```python
from build123d import *

# Parameters (mm, degrees)
F0_W      = 50.8
F0_H      = 76.2
F1_DEPTH  = 7.62
F2_R      = 18.7529717457
F3_DEPTH  = 5.08
F4_R      = 5.07999
F7_DEPTH  = 2.54
F8_W      = 50.2787431046
F8_H      = 6.6451809329
F9_DEPTH  = 2.286
F10_W     = 73.914
F10_H     = 6.6451809329
F11_DEPTH = 2.286
F12_W     = 48.514
F12_H     = 6.6451809329
F13_DEPTH = 2.286
F14_R     = 3.4596539052
F15_DEPTH = 25.4


# Not quite as in the source:
# - a fillet or chamfer is up to 0.001 mm smaller than in the source, because OpenCascade refuses the exact size


with BuildPart() as f1:
    # F0 (on Top) → F1 (new body)
    with BuildSketch(Plane.XY):
        with Locations((0.3819083795, -6.0587156958)):
            Rectangle(F0_W, F0_H)
    extrude(amount=F1_DEPTH)

    # F2 (on face) → F3 (join)
    with BuildSketch(Plane.XY.offset(7.62)):
        Circle(F2_R)
    extrude(amount=F3_DEPTH)

    # F4 (radius 5.08 in the source; OpenCascade refuses exactly that, so slightly less here)
    f4_edges = [f1.edges().sort_by_distance(p)[0] for p in [
        (-18.752972, 0, 12.7),
    ]]
    fillet(f4_edges, radius=F4_R)

    # F5 (on face) + F6 (on face) → F7 (join)
    with BuildSketch(Plane.XY.offset(7.62)):
        with BuildLine():
            ThreePointArc((-17.8012941845, -5.8981246722), (-18.7253311698, -1.0178024727), (-18.33570835, 3.9339228004))
            Line((-18.33570835, 3.9339228004), (-25.0180916205, 0.604446249))
            Line((-25.0180916205, 0.604446249), (-25.0180916205, -2.1975415816))
            Line((-25.0180916205, -2.1975415816), (-17.8012941845, -5.8981246722))
        make_face()
        with BuildLine():
            Line((-0.56613778, 26.5454184264), (-4.6479069665, 18.1678537567))
            ThreePointArc((-4.6479069665, 18.1678537567), (-0.450512239, 18.7475595216), (3.7698827091, 18.3701370069))
            Line((3.7698827091, 18.3701370069), (-0.56613778, 26.5454184264))
        make_face()
        with BuildLine():
            Line((18.8934579492, 18.5859743506), (10.2606709283, 15.6968971901))
            ThreePointArc((10.2606709283, 15.6968971901), (13.4651875999, 13.0523052444), (16.0087319261, 9.7670083143))
            Line((16.0087319261, 9.7670083143), (18.8934579492, 18.5859743506))
        make_face()
        with BuildLine():
            Line((25.7819083795, -1.3151803242), (25.7819083795, -0.2086242448))
            Line((25.7819083795, -0.2086242448), (18.4334550561, 3.4469818664))
            ThreePointArc((18.4334550561, 3.4469818664), (18.6729217202, 1.7308794659), (18.7529717457, 0))
            ThreePointArc((18.7529717457, 0), (18.5619015059, -2.6701613771), (17.9925843387, -5.2859112847))
            Line((17.9925843387, -5.2859112847), (25.7819083795, -1.3151803242))
        make_face()
        with BuildLine():
            ThreePointArc((15.6345242212, -10.3554624074), (12.4475757879, -14.0261115887), (8.4242275529, -16.7542931642))
            Line((8.4242275529, -16.7542931642), (18.9255586046, -20.1893288404))
            Line((18.9255586046, -20.1893288404), (15.6345242212, -10.3554624074))
        make_face()
        with BuildLine():
            ThreePointArc((4.5489366376, -18.1928866528), (-0.6058031571, -18.7431841433), (-5.7142487726, -17.8611676623))
            Line((-5.7142487726, -17.8611676623), (-0.3793946235, -28.119046241))
            Line((-0.3793946235, -28.119046241), (4.5489366376, -18.1928866528))
        make_face()
        with BuildLine():
            ThreePointArc((-8.8478629176, -16.5344873245), (-13.0678043341, -13.4501464371), (-16.2725260484, -9.3208822167))
            Line((-16.2725260484, -9.3208822167), (-19.8348792175, -20.2114386703))
            Line((-19.8348792175, -20.2114386703), (-8.8478629176, -16.5344873245))
        make_face()
    with BuildSketch(Plane.XY.offset(7.62)):
        with BuildLine():
            Line((-10.5754289904, 15.4865829337), (-19.9908912182, 18.6000298709))
            Line((-19.9908912182, 18.6000298709), (-16.5623554019, 8.7955859859))
            ThreePointArc((-16.5623554019, 8.7955859859), (-13.9752350774, 12.5046692809), (-10.5754289904, 15.4865829337))
        make_face()
    extrude(amount=F7_DEPTH)

    # F8 (on face) → F9 (cut)
    with BuildSketch(Plane(origin=(0, 32.0412843042, 0), x_dir=(-1, 0, 0), z_dir=(0, 1, 0))):
        with Locations((-0.6425368272, 3.8051904665)):
            Rectangle(F8_W, F8_H)
    extrude(amount=-F9_DEPTH, mode=Mode.SUBTRACT)

    # F10 (on face) → F11 (cut)
    with BuildSketch(Plane.YZ.offset(25.7819083795)):
        with Locations((-7.2017156958, 3.8051904665)):
            Rectangle(F10_W, F10_H)
    extrude(amount=-F11_DEPTH, mode=Mode.SUBTRACT)

    # F12 (on face) → F13 (cut)
    with BuildSketch(Plane.XZ.offset(44.1587156958)):
        with Locations((-0.7610916205, 3.8051904665)):
            Rectangle(F12_W, F12_H)
    extrude(amount=-F13_DEPTH, mode=Mode.SUBTRACT)

    # F14 (on face) → F15 (cut)
    with BuildSketch(Plane.XY.offset(7.62)):
        with Locations((0, -35.2311357856)):
            Circle(F14_R)
    extrude(amount=-F15_DEPTH, mode=Mode.SUBTRACT)


solid = f1.part
```
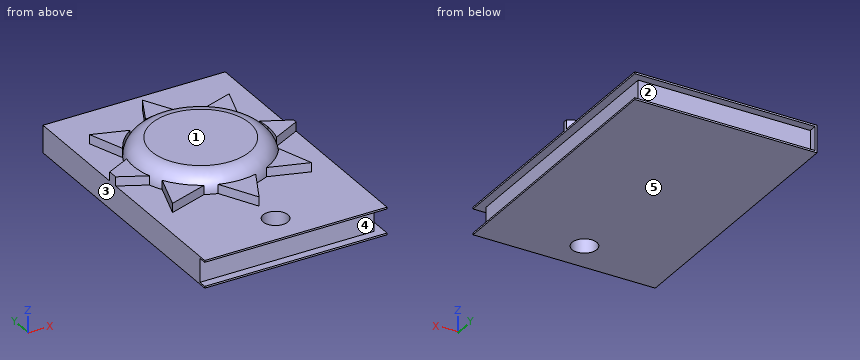
The model under review builds one solid part; all positions refer to its coordinate system, in mm. Face numbers are marked on the shaded views. A direction names the side the tool comes from. Round coordinates to 2 decimals unless told otherwise and drop trailing zeros. Order: outer loops, then holes, each group sorted by start corner. A loop starts at its lowest first (then second) coordinate and runs counter-clockwise, first axis right, second up. Notation, with made-up numbers: (63.5, 78) -> (110.5, 78) arc R35 ccw to (110.5, 111) -> close; hole circle Ø10 at (75, -12). An arc over 180 degrees is marked (long way). Use a Markdown table: item, result.
Q1. For line 1 (Y direction, x = 0, z = 6); line 2 (Z direction, x = -13, y = -33); line 3 (X direction, y = 22.5, z = 2), list the stretches that pass through material, from the lowest coordinate up.
Values:
| item | result |
|---|---|
| line 1 | y = -41.87 to -38.69, -31.77 to 29.76 |
| line 2 | z = 0 to 7.62 |
| line 3 | x = -25.02 to 23.5 |
Q2. Clearance check with flat-ended pins moving along their axes: P1, Ø7.5, axis at x = -17, y = 15, coming from the +Z side; P2, Ø1, axis at y = -22.5, z = 10, coming from the -X side; P3, Ø11, axis at x = 16, y = -14.5, coming from the +Z side; P4, Ø5.5, axis at x = 0, y = -35.23, coming from the -Z side. State where each tip first meets the part, or that it passes through.
Values:
| item | result |
|---|---|
| P1 | stops at z = 10.16 |
| P2 | stops at x = -3.56 |
| P3 | stops at z = 12.09 |
| P4 | passes through |
Q3. Tool access review of the marked faces 4 and 5: name each direction out of +Z, -Z, +X, -X, +Y, -Y from which nothing blocks a thin tool from reaching the whole face with its end or side.
Values:
| item | result |
|---|---|
| face 4 | +X, -X, -Y |
| face 5 | -Z, +X, -X, +Y, -Y |
Q4. We need section A-A on x = 20. Write out the cut boundary in (y, z), then the cut area to 3 significant figures.
Values:
| item | result |
|---|---|
| outline | (-44.16, 0) -> (32.04, 0) -> (32.04, 0.48) -> (29.76, 0.48) -> (29.76, 7.13) -> (32.04, 7.13) -> (32.04, 7.62) -> (2.67, 7.62) -> (2.67, 10.16) -> (-4.26, 10.16) -> (-4.26, 7.62) -> (-44.16, 7.62) -> (-44.16, 7.13) -> (-41.87, 7.13) -> (-41.87, 0.48) -> (-44.16, 0.48) -> close |
| area | 568 mm^2 |
Q5. Mouldability with a two-part tool opening along Z and no side actions: class the marked faces 1, 2 and 3 as +Z half, -Z half, draft (parallel to the pull), parting line (faces both ways), or undercut.
Values:
| item | result |
|---|---|
| face 1 | +Z half |
| face 2 | undercut |
| face 3 | draft |
